Model file for the job. Use its own axes, mm. Face numbers are marked on the shaded views. A direction names the side the tool comes from. Give positions to 0.01 mm unless a question says otherwise; leave off trailing zeros. Answer as CSV lines item,"result". Start each with the question number.
Item 1: Pin check, flat tips, straight feed: pin 1 (1 mm diameter, centred on y = 5.5, z = 2, fed in from +X); pin 2 (4 mm diameter, centred on y = -1, z = -1, fed in from -X); pin 3 (10 mm diameter, centred on y = 4, z = 8.5, fed in from -X); pin 4 (6.5 mm diameter, centred on x = 13.5, y = 2, fed in from -Z). Stop position of each tip, or through.
Item 2: Saw through at A-A on y = -6.75. State how many separate pieces and enclosed holes the cut face has, plus the area to 3 significant figures.
Item 3: Drill centre lines: L1, parallel to Y at x = 21.25, z = 0 (3 decimals); L2, parallel to X at y = -8.75, z = 5.75; L3, parallel to X at y = 1.75, z = 6.5. Where is each one in solid material? Low to high. Write a range as from..to.
Item 4: Tool access for the marked faces 1, 2 and 3: list every direction of +Z, -Z, +X, -X, +Y, -Y with a clear straight run to the whole face (end or side of a thin tool).
Item 5: Pull direction Z, two halves, no side cores. Call the marked faces 4, 5 and 6: pulls with the +Z half, pulls with the -Z half, needs draft (parallel to the pull), parting line crosses it, or undercut.
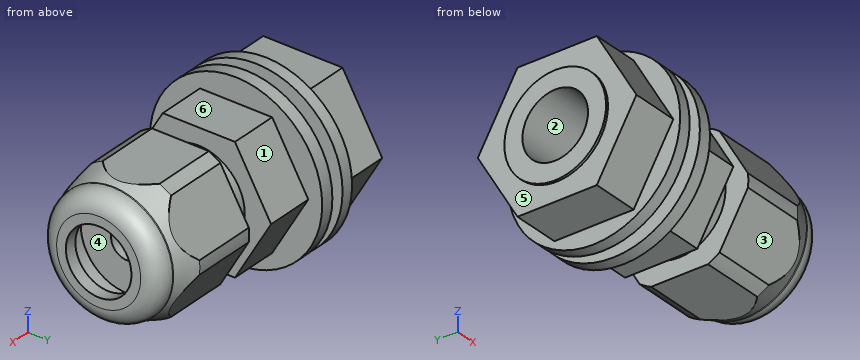
from build123d import *

# Parameters (mm, degrees)
SKETCH1_R           = 6.2
BOSS_EXTRUDE1_DEPTH = 10.8
BOSS_EXTRUDE2_DEPTH = 5.85
SKETCH3_R           = 5.6
BOSS_EXTRUDE3_DEPTH = 11.35
SKETCH4_R           = 10.5
BOSS_EXTRUDE4_DEPTH = 1.6
SKETCH5_R           = 10.5
BOSS_EXTRUDE5_DEPTH = 7.3
SKETCH6_R           = 13.375
CUT_EXTRUDE1_DEPTH  = 5.8
SKETCH7_R           = 4
CUT_EXTRUDE2_DEPTH  = 16.5
SKETCH8_R           = 1.9
CUT_EXTRUDE3_DEPTH  = 11.5
SKETCH10_R          = 12.625
CUT_EXTRUDE4_DEPTH  = 12.85


with BuildPart() as part:
    # Sketch1 → Boss-Extrude1 (new body)
    with BuildSketch(Plane(origin=(0, 0, 0), x_dir=(0, 0, -1), z_dir=(1, 0, 0))):
        with Locations(Location((0, 0, 0), (0, 0, 180))):
            Circle(SKETCH1_R)
    extrude(amount=BOSS_EXTRUDE1_DEPTH)

    # Sketch2 → Boss-Extrude2 (add)
    with BuildSketch(Plane(origin=(10.8, 0, 0), x_dir=(0, 0, -1), z_dir=(1, 0, 0))):
        Polygon((0, -8.804591605), (7.625, -4.402295803), (7.625, 4.402295803), (0, 8.804591605), (-7.625, 4.402295803), (-7.625, -4.402295803), align=None)
    extrude(amount=BOSS_EXTRUDE2_DEPTH)

    # Sketch3 → Boss-Extrude3 (add)
    with BuildSketch(Plane(origin=(16.65, 0, 0), x_dir=(0, 0, -1), z_dir=(1, 0, 0))):
        Circle(SKETCH3_R)
    extrude(amount=BOSS_EXTRUDE3_DEPTH)

    # Sketch4 → Boss-Extrude4 (add)
    with BuildSketch(Plane.ZY.offset(-10.8)):
        Circle(SKETCH4_R)
    extrude(amount=BOSS_EXTRUDE4_DEPTH)

    # Sketch5 → Boss-Extrude5 (add)
    with BuildSketch(Plane.ZY.offset(-7.6)):
        Circle(SKETCH5_R)
    extrude(amount=BOSS_EXTRUDE5_DEPTH)

    # Sketch6 → Cut-Extrude1 (cut)
    with BuildSketch(Plane.ZY.offset(-0.3)):
        Circle(SKETCH6_R)
        Polygon((0, -9.670617009), (8.375, -4.835308504), (8.375, 4.835308504), (0, 9.670617009), (-8.375, 4.835308504), (-8.375, -4.835308504), align=None, mode=Mode.SUBTRACT)
    extrude(amount=-CUT_EXTRUDE1_DEPTH, mode=Mode.SUBTRACT)

    # Sketch7 → Cut-Extrude2 (cut)
    with BuildSketch(Plane.ZY):
        Circle(SKETCH7_R)
    extrude(amount=-CUT_EXTRUDE2_DEPTH, mode=Mode.SUBTRACT)

    # Sketch8 → Cut-Extrude3 (cut)
    with BuildSketch(Plane(origin=(28, 0, 0), x_dir=(0, 0, -1), z_dir=(1, 0, 0))):
        Circle(SKETCH8_R)
    extrude(amount=-CUT_EXTRUDE3_DEPTH, mode=Mode.SUBTRACT)

    # Sketch9 → Revolve1 (revolve)
    with BuildSketch(Plane.XY, mode=Mode.PRIVATE) as revolve1_sk:
        with BuildLine():
            Line((19.55, 8.375), (27.3, 8.375))
            Line((27.3, 8.375), (30.05, 7.325))
            Line((30.05, 7.325), (30.2, 7.325))
            ThreePointArc((30.2, 7.325), (31.755634919, 6.680634919), (32.4, 5.125))
            Line((32.4, 5.125), (32.4, 4))
            Line((32.4, 4), (30.9, 4))
            Line((30.9, 4), (30.9, 5.125))
            ThreePointArc((30.9, 5.125), (30.760875721, 5.460875721), (30.425, 5.6))
            Line((30.425, 5.6), (19.55, 5.6))
            Line((19.55, 5.6), (19.55, 8.375))
        make_face()
    revolve(revolve1_sk.sketch.rotate(Axis((0, 0, 0), (1, 0, 0)), 90), axis=Axis((0, 0, 0), (1, 0, 0)))

    # Sketch10 → Cut-Extrude4 (cut)
    with BuildSketch(Plane(origin=(32.4, 0, 0), x_dir=(0, 0, -1), z_dir=(1, 0, 0))):
        Circle(SKETCH10_R)
        Polygon((7.625, -4.402295803), (7.625, 4.402295803), (0, 8.804591605), (-7.625, 4.402295803), (-7.625, -4.402295803), (0, -8.804591605), align=None, mode=Mode.SUBTRACT)
    extrude(amount=-CUT_EXTRUDE4_DEPTH, mode=Mode.SUBTRACT)


solid = part.part
Responses:
1,pin 1,"x = 32.39"
1,pin 2,"x = 16.5"
1,pin 3,"x = 0"
1,pin 4,"z = -10.5"
2,separate pieces,"3"
2,enclosed holes,"0"
2,area,"232 mm2"
3,L1,"-8.375..-1.9, 1.9..8.375"
3,L2,"6.1..7.6, 9.2..10.8"
3,L3,"0.3..7.6, 9.2..16.65, 19.55..31.7"
4,face 1,"+Z, +X, +Y"
4,face 2,"-X"
4,face 3,"-Z, +X, -Y"
5,face 4,"undercut"
5,face 5,"needs draft"
5,face 6,"pulls with the +Z half"
